from build123d import *

# Parameters (mm, degrees)
SKETCH4_W           = 10
SKETCH4_H           = 3
BOSS_EXTRUDE2_DEPTH = 2
SKETCH5_W           = 4
SKETCH5_H           = 3
BOSS_EXTRUDE3_DEPTH = 3
SKETCH6_W           = 2
SKETCH6_H           = 3
BOSS_EXTRUDE4_DEPTH = 6
SKETCH7_W           = 2
SKETCH7_H           = 3
BOSS_EXTRUDE5_DEPTH = 2
SKETCH8_W           = 2
SKETCH8_H           = 3
BOSS_EXTRUDE6_DEPTH = 2


with BuildPart() as part:
    # Sketch4 → Boss-Extrude2 (new body)
    with BuildSketch(Plane.XY):
        with Locations((-112.42360649, 35.715193832)):
            Rectangle(SKETCH4_W, SKETCH4_H)
    extrude(amount=BOSS_EXTRUDE2_DEPTH)

    # Sketch5 → Boss-Extrude3 (add)
    with BuildSketch(Plane(origin=(0, 0, 0), x_dir=(-1, 0, 0), z_dir=(0, 0, -1))):
        with Locations((114.42360649, 35.715193832)):
            Rectangle(SKETCH5_W, SKETCH5_H)
        with Locations((110.42360649, 35.715193832)):
            Rectangle(SKETCH5_W, SKETCH5_H)
    extrude(amount=BOSS_EXTRUDE3_DEPTH)

    # Sketch6 → Boss-Extrude4 (add)
    with BuildSketch(Plane.XY.offset(2)):
        with Locations((-108.42360649, 35.715193832)):
            Rectangle(SKETCH6_W, SKETCH6_H)
        with Locations((-116.42360649, 35.715193832)):
            Rectangle(SKETCH6_W, SKETCH6_H)
    extrude(amount=BOSS_EXTRUDE4_DEPTH)

    # Sketch7 → Boss-Extrude5 (add)
    with BuildSketch(Plane(origin=(-115.42360649, 0, 0), x_dir=(0, 0, -1), z_dir=(1, 0, 0))):
        with Locations((-7, 35.715193832)):
            Rectangle(SKETCH7_W, SKETCH7_H)
    extrude(amount=BOSS_EXTRUDE5_DEPTH)

    # Sketch8 → Boss-Extrude6 (add)
    with BuildSketch(Plane.ZY.offset(109.42360649)):
        with Locations((7, 35.715193832)):
            Rectangle(SKETCH8_W, SKETCH8_H)
    extrude(amount=BOSS_EXTRUDE6_DEPTH)


solid = part.part
Work out the finished part from the listing and answer in its coordinate system (mm). A direction names the side the tool comes from. Round coordinates to 2 decimals unless told otherwise and drop trailing zeros. Loops run counter-clockwise (first coordinate to the right, second up) from the corner with the lowest first, then second, coordinate; pieces in that order, holes last. Notation, with made-up numbers: (-27, 51) -> (-1, 51) arc R27 ccw to (-1, 90) -> close; hole circle Ø1 at (72.25, 74.25). An arc over 180 degrees is marked (long way). Use one line per item in the form item = value.
(1) For a pull along X with two mould halves and no side action, classify faces 1 (the flat face through (-114, 36, 6)), 2 (the flat face through (-108.424, 36, -1)), 3 (the flat face through (-108, 36, 0)), 4 (the flat face through (-117.424, 36, 4)) as released by +X, released by -X, zero draft, split by the parting line, or undercut.
Answer list:
face_1 = undercut
face_2 = released by +X
face_3 = zero draft
face_4 = released by -X
(2) Find section C-C on y = 34.75. Give the vertices of the cut face in (x, z), then the cut area to 3 significant figures.
Answer list:
outline = (-117.42, 0) -> (-116.42, 0) -> (-116.42, -3) -> (-108.42, -3) -> (-108.42, 0) -> (-107.42, 0) -> (-107.42, 8) -> (-111.42, 8) -> (-111.42, 6) -> (-109.42, 6) -> (-109.42, 2) -> (-115.42, 2) -> (-115.42, 6) -> (-113.42, 6) -> (-113.42, 8) -> (-117.42, 8) -> close
area = 76.0 mm2
(3) Find section D-D on x = -113. Give the vertices of the cut face in (y, z), then the cut area to 3 significant figures.
Answer list:
outline = (34.22, -3) -> (37.22, -3) -> (37.22, 2) -> (34.22, 2) -> close
area = 15.0 mm2
(4) Find section A-A on x = -109.75. Give the vertices of the cut face in (y, z).
Answer list:
outline = (34.22, -3) -> (37.22, -3) -> (37.22, 2) -> (34.22, 2) -> close; (34.22, 6) -> (37.22, 6) -> (37.22, 8) -> (34.22, 8) -> close
(5) Straight lines are drawn through the part: line 1 (X direction, y = 35.75, z = 4.25); line 2 (Z direction, x = -114.25, y = 37.05); line 3 (X direction, y = 34.5, z = -2). For each, find the intervals that lie inside material, in ascending order.
Answer list:
line_1 = -117.42 to -115.42, -109.42 to -107.42
line_2 = -3 to 2, 6 to 8
line_3 = -116.42 to -108.42
(6) A tool of negligible diameter and unlimited length cuts with its end or side. For faces 5 (the flat face through (-111.424, 36, 7)), 6 (the flat face through (-117, 36, 0)), 7 (the flat face through (-115.424, 36, 4)), from which of +Z, -Z, +X, -X, +Y, -Y can it reach the whole face along a straight path? Write none if from no direction.
Answer list:
face_5 = +Z, +Y, -Y
face_6 = -Z, -X, +Y, -Y
face_7 = +Y, -Y
(7) A flat-ended cylindrical pin translates along its axis: P1, Ø0.5, axis at x = -117, y = 36.5, coming from the -Z side. Find the tip coordinate at first contact, or state that the pin passes through.
Answer list:
P1 = 0
(8) Find section B-B on z = 4.5. Give the vertices of the cut face in (x, y).
Answer list:
outline = (-117.42, 34.22) -> (-115.42, 34.22) -> (-115.42, 37.22) -> (-117.42, 37.22) -> close; (-109.42, 34.22) -> (-107.42, 34.22) -> (-107.42, 37.22) -> (-109.42, 37.22) -> close
